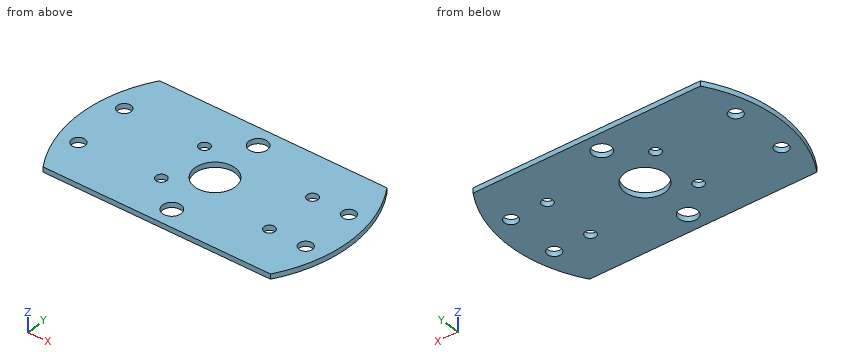
Autodesk Inventor part; units mm, degrees
ref_plane "YZ Plane" through (0, 0, 0) normal (1, 0, 0) x (0, 1, 0)
ref_plane "XZ Plane" through (0, 0, 0) normal (0, 1, 0) x (-1, 0, 0)
ref_plane "XY Plane" through (0, 0, 0) normal (0, 0, 1) x (1, 0, 0)
sketch "スケッチ1" plane through (0, 0, 0) normal (0, 0, 1) x (1, 0, 0)
  point P0 (0, 0)
ref_plane "作業平面1" through (242.6146, -15.2304, -10) normal (0, 0, 1) x (1, 0, 0)
sketch "スケッチ2" plane through (242.6146, -15.2304, -10) normal (0, 0, 1) x (1, 0, 0)
  line L0 (-33.6666, -21.6) -> (33.6666, -21.6)
  arc A0 (33.6666, -21.6) -> (33.6666, 21.6) centre (0, 0) ccw
  line L1 (33.6666, 21.6) -> (-33.6666, 21.6)
  arc A1 (-33.6666, 21.6) -> (-33.6666, -21.6) centre (0, 0) ccw
  circle A2 centre (33.25, -8) radius 2
  circle A3 centre (33.25, 8) radius 2
  circle A4 centre (22.5, 8) radius 1.6
  circle A5 centre (22.5, -8) radius 1.6
  line L2 (-4.9746, -0.5032) -> (-4.9749, 0.5004)
  arc A6 (-4.9746, -0.5032) -> (-4.9749, 0.5004) centre (0, 0) ccw
  circle A7 centre (-33.25, 8) radius 2
  circle A8 centre (-9.5, -8) radius 1.6
  circle A9 centre (-9.5, 8) radius 1.6
  circle A10 centre (-33.25, -9) radius 2
  circle A11 centre (0, 0) radius 6
  circle A12 centre (0, 16) radius 2.75
  circle A13 centre (0, -16) radius 2.75
  point P0 (-242.6146, 15.2304)
  dimension "d0" = 12
extrude "押し出し1" add sketch "スケッチ2" along normal blind 1.5 contours A1 L1 A0 L0
Input: part model. Units: mm. Frame: model coordinates. Give positions to 0.01 mm unless a question says otherwise; leave off trailing zeros. Order: outer loops, then holes, each group sorted by start corner. A loop starts at its lowest first (then second) coordinate and runs counter-clockwise, first axis right, second up.
Q1. Ray query, probe 1 along X at (y, z) = (-23, -9.8); probe 2 along X at (y, z) = (-9, -9.3); probe 3 along X at (y, z) = (-6, -8.7). Return the intervals inside material, ascending.
Checked values:
probe 1: x = 203.38 to 207.79, 210.94 to 231.53, 234.7 to 263.53, 266.7 to 273.88, 277.85 to 281.85
probe 2: x = 203.1 to 208.43, 210.3 to 274.93, 276.8 to 282.13
probe 3: x = 203.69 to 207.79, 210.94 to 232.09, 234.14 to 264.09, 266.14 to 274.29, 277.44 to 281.54
Q2. Section A-A on y = -19.5. Output: boundary loops of the cut face in (x, z), and give its area (3 significant figures).
Checked values:
outline: (202.84, -10) - (238.4, -10) - (238.4, -8.5) - (202.84, -8.5) - close; (246.83, -10) - (282.39, -10) - (282.39, -8.5) - (246.83, -8.5) - close
area: 107 mm2
Q3. Section C-C on z = -9.05. State how many separate pieces and enclosed holes the cut face has, and give its area (3 significant figures).
Checked values:
separate pieces: 1
enclosed holes: 11
area: 3,040 mm2
Q4. Section B-B on x = 210. Output: boundary loops of the cut face in (y, z).
Checked values:
outline: (-36.83, -10) - (-26.13, -10) - (-26.13, -8.5) - (-36.83, -8.5) - close; (-22.33, -10) - (-9.13, -10) - (-9.13, -8.5) - (-22.33, -8.5) - close; (-5.33, -10) - (6.37, -10) - (6.37, -8.5) - (-5.33, -8.5) - close
Q5. Section D-D on y = -33. Output: boundary loops of the cut face in (x, z), and give its area (3 significant figures).
Checked values:
outline: (206.78, -10) - (240.51, -10) - (240.51, -8.5) - (206.78, -8.5) - close; (244.72, -10) - (278.45, -10) - (278.45, -8.5) - (244.72, -8.5) - close
area: 101 mm2
